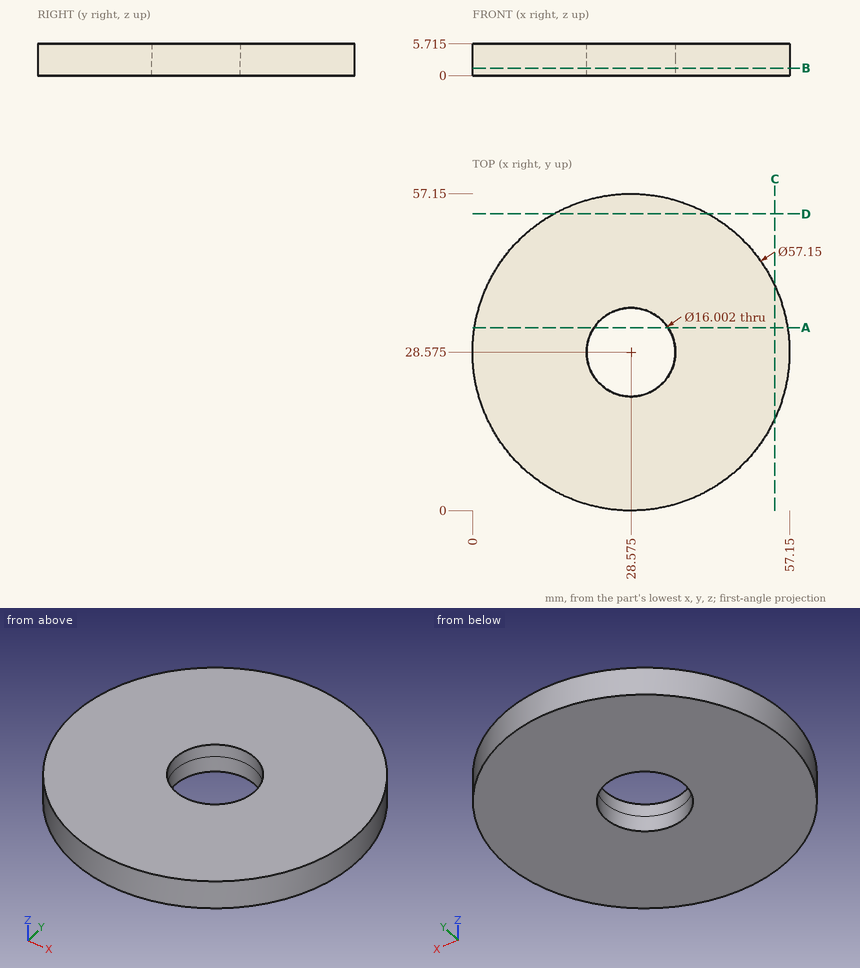
Source: three-view drawing plus pictorial views. Frame: mm from the lowest corner of the part. Give positions to 0.01 mm unless a question says otherwise; leave off trailing zeros. Write each loop counter-clockwise with the first axis right and the second up, starting at its lowest first coordinate (ties: lowest second). Pieces come first, ordered by that corner, then holes. Notation, with made-up numbers: (-2.75, 12.5) -> (44.25, 12.5) arc R17 ccw to (44.25, 43.5) -> close; hole circle Ø3 at (-3.5, 50.5). An arc over 180 degrees is marked (long way). Answer in a Markdown table with one row per item.
(1) Section query A-A on y = 33. Return loops of the section in (x, z) (3 decimals), then the cut area to 3 significant figures.
Answers below:
| item | result |
|---|---|
| outline | (0.345, 0) -> (21.909, 0) -> (21.909, 5.715) -> (0.345, 5.715) -> close; (35.241, 0) -> (56.805, 0) -> (56.805, 5.715) -> (35.241, 5.715) -> close |
| area | 246 mm^2 |
(2) Section query B-B on z = 1.35. Return loops of the section in (x, y) (3 decimals).
Answers below:
| item | result |
|---|---|
| outline | circle Ø57.15 at (28.575, 28.575); hole circle Ø16.002 at (28.575, 28.575) |
(3) Pin query (flat end, axial travel): pin 1 (1 mm diameter, centred on x = 31, z = 4, fed in from +Y); pin 2 (1 mm diameter, centred on x = 10.5, z = 2.5, fed in from +Y). Return the tip coordinate at first contact, or that it passes through.
Answers below:
| item | result |
|---|---|
| pin 1 | y = 57.09 |
| pin 2 | y = 51.11 |
(4) Section query D-D on y = 53.5. Return loops of the section in (x, z) (3 decimals).
Answers below:
| item | result |
|---|---|
| outline | (14.601, 0) -> (42.549, 0) -> (42.549, 5.715) -> (14.601, 5.715) -> close |
(5) Section query C-C on x = 54.5. Return loops of the section in (y, z) (3 decimals), then the cut area to 3 significant figures.
Answers below:
| item | result |
|---|---|
| outline | (16.557, 0) -> (40.593, 0) -> (40.593, 5.715) -> (16.557, 5.715) -> close |
| area | 137 mm^2 |
(6) Ray query, line 1 along Y through (x, z) = (28, 4.7); line 2 along X through (y, z) = (23, 5.1); line 3 along Y through (x, z) = (55, 5.5). Return the intervals inside material, ascending. Write a range as [from, to].
Answers below:
| item | result |
|---|---|
| line 1 | [0.01, 20.59], [36.56, 57.14] |
| line 2 | [0.55, 22.84], [34.31, 56.6] |
| line 3 | [17.7, 39.45] |
